Part model, mm, in its own coordinate system. A direction names the side the tool comes from. Coordinates: 2 decimals unless noted, no trailing zeros. Write each loop counter-clockwise with the first axis right and the second up, starting at its lowest first coordinate (ties: lowest second). Pieces come first, ordered by that corner, then holes. Notation, with made-up numbers: M 57.5,62.25 L 71.5,62.25 A10 cw 71.5,77.25 Z; hole C -35,-19.75 d3. An arc over 180 degrees is marked long. Use a Markdown table: item, result. Add a question column.
Q1. Wall check: L1, parallel to X at y = -13, z = -189; L2, parallel to Z at x = 6, y = -2.5; L3, parallel to Z at x = -249, y = -2.5. Give the ranges that are in metal, low to high. Write a range as from..to.
Q2. Slice it at B-B on y = -10.5. Write the cut outline in (x, z).
Q3. Mould opens along Z. For faces 1 (the flat face through (-265, -13, -15)), 2 (the flat face through (-30, -13, -60)), 3 (the flat face through (-333.691, -12.818, -234.486)) say: released by +Z, released by -Z, zero draft, split by the parting line, or undercut.
Q4. Slice it at A-A on z = -220. Write the cut outline in (x, y), then the cut area to 3 significant figures.
Q5. Tool access for faces 4 (the flat face through (-42, -26, -75)), 5 (the flat face through (264, -13, -15)), 6 (the flat face through (0, -13, -45)): list every direction of +Z, -Z, +X, -X, +Y, -Y with a clear straight run to the whole face (end or side of a thin tool).
Q6. Pin check, flat tips, straight feed: pin 1 Ø8 at (x, y) = (2.5, -19.5) entering from -Z; pin 2 Ø5 at (y, z) = (-2.5, -257) entering from -X; pin 3 Ø12 at (x, y) = (-357, -22.5) entering from -Z. Stop position of each tip, or through.
Q7. Slice it at C-C on z = -160. Write the cut outline in (x, y).
Q8. Slice it at D-D on x = 392.5. Write the cut outline in (y, z).
from build123d import *

# Parameters (mm, degrees)
F1_DEPTH = 26


with BuildPart() as f1:
    # F0 (on Front) → F1 (new body)
    with BuildSketch(Plane.XZ):
        with BuildLine():
            ThreePointArc((522.115478, -370), (526.65902, -367.087157), (525.908713, -361.74249))
            Line((525.908713, -361.74249), (245.312642, -35))
            ThreePointArc((245.312642, -35), (243.49537, -22.055015), (254.5, -15))
            Line((254.5, -15), (274.5, -15))
            Line((274.5, -15), (274.5, 0))
            Line((274.5, 0), (-274.5, 0))
            Line((-274.5, 0), (-274.5, -15))
            Line((-274.5, -15), (-254.5, -15))
            ThreePointArc((-254.5, -15), (-243.49537, -22.055015), (-245.312642, -35))
            Line((-245.312642, -35), (-525.908713, -361.74249))
            ThreePointArc((-525.908713, -361.74249), (-526.65902, -367.087157), (-522.115478, -370))
            Line((-522.115478, -370), (-500.930536, -370))
            ThreePointArc((-500.930536, -370), (-494.044191, -368.777067), (-488, -365.257826))
            Line((-488, -365.257826), (-175, -100))
            ThreePointArc((-175, -100), (-103.279947, -82.867809), (-30, -74.662483))
            Line((-30, -74.662483), (-30, -45))
            Line((-30, -45), (30, -45))
            Line((30, -45), (30, -74.662483))
            ThreePointArc((30, -74.662483), (103.279947, -82.867809), (175, -100))
            Line((175, -100), (488, -365.257826))
            ThreePointArc((488, -365.257826), (494.044191, -368.777067), (500.930536, -370))
            Line((500.930536, -370), (522.115478, -370))
        make_face()
    extrude(amount=F1_DEPTH)


solid = f1.part
Recorded:
| question | item | result |
|---|---|---|
| 1 | L1 | -377.56..-280.02, 280.02..377.56 |
| 1 | L2 | -45..0 |
| 1 | L3 | -162.71..-39.29, -16.32..0 |
| 2 | outline | M -525.91,-361.74 A5 ccw -522.12,-370 L -500.93,-370 A20 ccw -488,-365.26 L -175,-100 A600 cw -30,-74.66 L -30,-45 L 30,-45 L 30,-74.66 A600 cw 175,-100 L 488,-365.26 A20 ccw 500.93,-370 L 522.12,-370 A5 ccw 525.91,-361.74 L 245.31,-35 A12.11 cw 254.5,-15 L 274.5,-15 L 274.5,0 L -274.5,0 L -274.5,-15 L -254.5,-15 A12.11 cw -245.31,-35 Z |
| 3 | face 1 | undercut |
| 3 | face 2 | zero draft |
| 3 | face 3 | released by -Z |
| 4 | outline | M -404.18,-26 L -316.6,-26 L -316.6,0 L -404.18,0 Z; M 316.6,-26 L 404.18,-26 L 404.18,0 L 316.6,0 Z |
| 4 | area | 4,550 mm² |
| 5 | face 4 | +Z, -Z, +X, -X, -Y |
| 5 | face 5 | +X, +Y, -Y |
| 5 | face 6 | -Z, +Y, -Y |
| 6 | pin 1 | z = -45 |
| 6 | pin 2 | x = -438.11 |
| 6 | pin 3 | z = -259.32 |
| 7 | outline | M -352.66,-26 L -245.8,-26 L -245.8,0 L -352.66,0 Z; M 245.8,-26 L 352.66,-26 L 352.66,0 L 245.8,0 Z |
| 8 | outline | M -26,-284.32 L 0,-284.32 L 0,-206.39 L -26,-206.39 Z |
